from build123d import *

# Parameters (mm, degrees)
SKETCH1_W               = 20
SKETCH1_H               = 30
BOSS_EXTRUDE1_DEPTH     = 3
SKETCH2_W               = 5
SKETCH2_H               = 12
BOSS_EXTRUDE2_DEPTH     = 3
SKETCH3_R               = 7
SKETCH3_R_2             = 4
BOSS_EXTRUDE3_DEPTH     = 7
SKETCH4_R               = 4
BOSS_EXTRUDE4_DEPTH     = 1
CUT_EXTRUDE1_DEPTH      = 20.339079606
CUT_EXTRUDE1_DEPTH_BACK = 20.339079606
SKETCH5_R               = 3
SKETCH6_R               = 7
SKETCH6_R_2             = 4
BOSS_EXTRUDE6_DEPTH     = 7
SKETCH7_W               = 20
SKETCH7_H               = 3
BOSS_EXTRUDE7_DEPTH     = 19
SKETCH8_W               = 5
SKETCH8_H               = 3
BOSS_EXTRUDE8_DEPTH     = 12
CUT_EXTRUDE2_START      = -1.5
SKETCH10_R              = 4
CUT_EXTRUDE2_DEPTH      = 1.5
SKETCH12_W              = 3
SKETCH12_H              = 32
BOSS_EXTRUDE9_DEPTH     = 5


with BuildPart() as part:
    # Sketch1 → Boss-Extrude1 (new body)
    with BuildSketch(Plane(origin=(0, 0, 0), x_dir=(1, 0, 0), z_dir=(0, 1, 0))):
        Rectangle(SKETCH1_W, SKETCH1_H)
    boss_extrude1 = extrude(amount=BOSS_EXTRUDE1_DEPTH)

    # Sketch2 → Boss-Extrude2 (add)
    with BuildSketch(Plane.XZ):
        with Locations((0, -9)):
            Rectangle(SKETCH2_W, SKETCH2_H)
    boss_extrude2 = extrude(amount=BOSS_EXTRUDE2_DEPTH)

    # Sketch3 → Boss-Extrude3 (add)
    with BuildSketch(Plane(origin=(0, 3, 0), x_dir=(1, 0, 0), z_dir=(0, 1, 0))):
        with Locations(Location((0, 8, 0), (0, 0, 90))):
            Circle(SKETCH3_R)
        with Locations(Location((0, 8, 0), (0, 0, 270))):
            Circle(SKETCH3_R_2, mode=Mode.SUBTRACT)
    boss_extrude3 = extrude(amount=BOSS_EXTRUDE3_DEPTH)

    # Sketch4 → Boss-Extrude4 (add)
    with BuildSketch(Plane(origin=(0, 3, 0), x_dir=(1, 0, 0), z_dir=(0, 1, 0))):
        with Locations(Location((0, 8, 0), (0, 0, 270))):
            Circle(SKETCH4_R)
    boss_extrude4 = extrude(amount=BOSS_EXTRUDE4_DEPTH)

    # Sketch5 → Cut-Extrude1 (cut, two sides: drawn at the far end of the back side and taken through both)
    with BuildSketch(Plane(origin=(0, 3, 0), x_dir=(1, 0, 0), z_dir=(0, 1, 0)).offset(-CUT_EXTRUDE1_DEPTH_BACK)):
        with Locations(Location((0, -8.5, 0), (0, 0, 90))):
            Circle(SKETCH5_R)
    extrude(amount=CUT_EXTRUDE1_DEPTH + CUT_EXTRUDE1_DEPTH_BACK, mode=Mode.SUBTRACT)

    # Sketch6 → Boss-Extrude6 (add)
    # profile 1 of 2: a face of its own
    with BuildSketch(Plane(origin=(0, 3, 0), x_dir=(1, 0, 0), z_dir=(0, 1, 0))):
        Polygon((0, 15), (-10, 15), (-10, -1), (10, -1), (10, 15), align=None)
        with BuildLine():
            ThreePointArc((7, 8), (-4.949747468, 3.050252532), (0, 15))
            ThreePointArc((0, 15), (4.949747468, 12.949747468), (7, 8))
        make_face(mode=Mode.SUBTRACT)
    # profile 2 of 2: a face of its own
    with BuildSketch(Plane(origin=(0, 3, 0), x_dir=(1, 0, 0), z_dir=(0, 1, 0))):
        with Locations((0, 8)):
            Circle(SKETCH6_R)
        with Locations(Location((0, 8, 0), (0, 0, 270))):
            Circle(SKETCH6_R_2, mode=Mode.SUBTRACT)
    boss_extrude6 = extrude(amount=BOSS_EXTRUDE6_DEPTH)

    # Sketch7 → Boss-Extrude7 (add)
    with BuildSketch(Plane.XY.offset(15)):
        with Locations((0, 1.5)):
            Rectangle(SKETCH7_W, SKETCH7_H)
    extrude(amount=BOSS_EXTRUDE7_DEPTH)

    # Mirror3: Boss-Extrude1, Boss-Extrude2, Boss-Extrude3, Boss-Extrude4, Boss-Extrude6 across plane
    add(boss_extrude1.mirror(Plane.XY.offset(17)))
    add(boss_extrude2.mirror(Plane.XY.offset(17)))
    add(boss_extrude3.mirror(Plane.XY.offset(17)))
    add(boss_extrude4.mirror(Plane.XY.offset(17)))
    add(boss_extrude6.mirror(Plane.XY.offset(17)))

    # Sketch8 → Boss-Extrude8 (add)
    with BuildSketch(Plane(origin=(0, 0, 37), x_dir=(-1, 0, 0), z_dir=(0, 0, -1))):
        with Locations((0, -1.5)):
            Rectangle(SKETCH8_W, SKETCH8_H)
    extrude(amount=BOSS_EXTRUDE8_DEPTH)

    # Sketch10 → Cut-Extrude2 (cut)
    with BuildSketch(Plane(origin=(0, 4, 0), x_dir=(1, 0, 0), z_dir=(0, 1, 0)).offset(CUT_EXTRUDE2_START)):
        with Locations(Location((0, 8, 0), (0, 0, 270))):
            Circle(SKETCH10_R)
        with Locations(Location((0, -42, 0), (0, 0, 90))):
            Circle(SKETCH10_R)
    extrude(amount=CUT_EXTRUDE2_DEPTH, mode=Mode.SUBTRACT)

    # Sketch12 → Boss-Extrude9 (add)
    with BuildSketch(Plane(origin=(0, 3, 0), x_dir=(1, 0, 0), z_dir=(0, 1, 0))):
        with Locations((8.5, -17)):
            Rectangle(SKETCH12_W, SKETCH12_H)
        with Locations((-8.5, -17)):
            Rectangle(SKETCH12_W, SKETCH12_H)
    extrude(amount=BOSS_EXTRUDE9_DEPTH)


solid = part.part
Check sheet for the modelled part. Datum: model origin and axes. Units: mm. A direction names the side the tool comes from. Coordinates: 2 decimals unless noted, no trailing zeros. Write each loop counter-clockwise with the first axis right and the second up, starting at its lowest first coordinate (ties: lowest second). Pieces come first, ordered by that corner, then holes.
Item 1: Cross-section at C-C on y = 6.5. Record the boundary of the cut face in (x, z), then the cut area to 3 significant figures.
Numbers:
outline: (-10, -15) - (10, -15) - (10, 49) - (-10, 49) - close; hole (-7, 1) - (7, 1) - (7, 33) - (-7, 33) - close; hole circle Ø8 at (0, -8); hole circle Ø8 at (0, 42)
area: 731 mm2
Item 2: Depth check by flat-ended pin: pin 1 Ø1.5 at (x, z) = (8.5, 12) entering from +Y; pin 2 Ø4 at (x, z) = (2, 22) entering from +Y; pin 3 Ø3.5 at (y, z) = (-2, 40) entering from -X; pin 4 Ø5 at (x, z) = (0, 8.5) entering from -Y. Enter the tip coordinate at first touch or a pass-through.
Numbers:
pin 1: stops at y = 8
pin 2: stops at y = 3
pin 3: stops at x = -2.5
pin 4: passes through
Item 3: Mould release check, pull along Z, two halves, no side actions. Record for faces 1 (the face through (0, 6, 33)), 2 (the face through (0, 5, 49)), 3 (the face through (-0.1, 10, -3.6)): released by +Z, released by -Z, zero draft, split by the parting line, or undercut.
Numbers:
face 1: undercut
face 2: released by +Z
face 3: zero draft
Item 4: Scan lines: probe 1 along X at (y, z) = (2.3, 8.5); probe 2 along Z at (x, y) = (0.75, 2.75); probe 3 along Y at (x, z) = (4.75, -11). Record each from-to range of solid material in increasing order.
Numbers:
probe 1: x = -10 to -3, 3 to 10
probe 2: z = -15 to -11.93, -4.07 to 5.6, 11.4 to 38.07, 45.93 to 49
probe 3: y = 0 to 10
Item 5: Cross-section at D-D on z = 2. Record the boundary of the cut face in (x, y).
Numbers:
outline: (-10, 0) - (10, 0) - (10, 8) - (7, 8) - (7, 3) - (-7, 3) - (-7, 8) - (-10, 8) - close
Item 6: Access from +Z, -Z, +X, -X, +Y, -Y to the whole of each face (thin tool, end or side, straight path). Record for faces 4 (the face through (0, -1, -3)), 5 (the face through (-9, 8, 17)), 6 (the face through (2.5, -1, -9)), 7 (the face through (7, 5, 17)).
Numbers:
face 4: +X, -X, -Y
face 5: +X, -X, +Y
face 6: +Z, -Z, +X, -Y
face 7: +Y
Item 7: Cross-section at A-A on z = 8.5. Record the boundary of the cut face in (x, y), then the cut area to 3 significant figures.
Numbers:
outline: (-10, 0) - (-3, 0) - (-3, 3) - (-7, 3) - (-7, 8) - (-10, 8) - close; (3, 0) - (10, 0) - (10, 8) - (7, 8) - (7, 3) - (3, 3) - close
area: 72.0 mm2
Item 8: Cross-section at B-B on x = 0. Record the boundary of the cut face in (y, z).
Numbers:
outline: (-3, -15) - (10, -15) - (10, -12) - (2.5, -12) - (2.5, -4) - (10, -4) - (10, 1) - (3, 1) - (3, 5.5) - (0, 5.5) - (0, -3) - (-3, -3) - close; (-3, 25) - (0, 25) - (0, 11.5) - (3, 11.5) - (3, 33) - (10, 33) - (10, 38) - (2.5, 38) - (2.5, 46) - (10, 46) - (10, 49) - (-3, 49) - close
